Drawing for the job (mm, zero at the part's lowest x, y, z). Round coordinates to 2 decimals unless told otherwise and drop trailing zeros. Order: outer loops, then holes, each group sorted by start corner. A loop starts at its lowest first (then second) coordinate and runs counter-clockwise, first axis right, second up. Notation, with made-up numbers: (76, 6.5) -> (113, 6.5) arc R22 ccw to (113, 45.5) -> close; hole circle Ø7 at (63.5, 27.5). An arc over 180 degrees is marked (long way). Use CSV: the item, a comma, the result in double quotes.
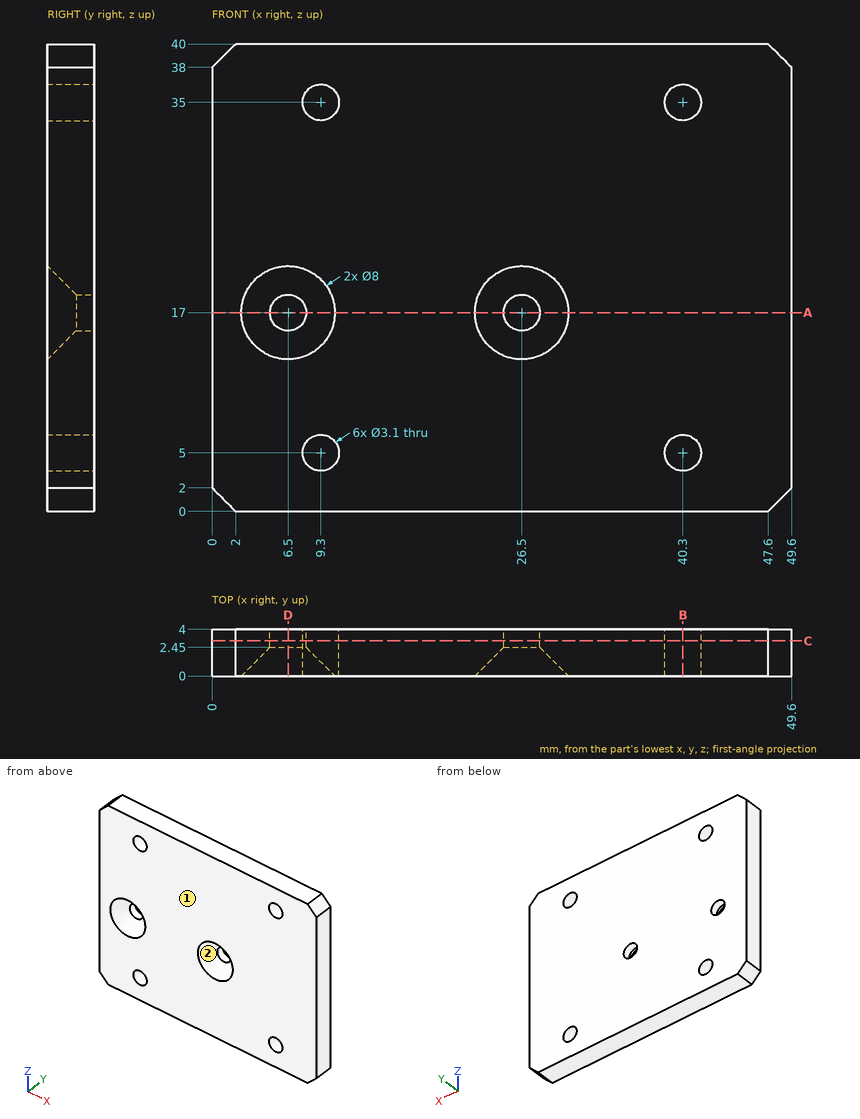
Q1. Cut at A-A (z = 17). Give the cut face in (x, y).
From the geometry:
outline,"(0, 0) -> (2.5, 0) -> (4.95, 2.45) -> (4.95, 4) -> (0, 4) -> close; (8.05, 2.45) -> (10.5, 0) -> (22.5, 0) -> (24.95, 2.45) -> (24.95, 4) -> (8.05, 4) -> close; (28.05, 2.45) -> (30.5, 0) -> (49.6, 0) -> (49.6, 4) -> (28.05, 4) -> close"
Q2. Cut at B-B (x = 40.3). Give the cut face in (y, z), plus the area to 3 significant figures.
From the geometry:
outline,"(0, 0) -> (4, 0) -> (4, 3.45) -> (0, 3.45) -> close; (0, 6.55) -> (4, 6.55) -> (4, 33.45) -> (0, 33.45) -> close; (0, 36.55) -> (4, 36.55) -> (4, 40) -> (0, 40) -> close"
area,"135 mm²"
Q3. Mould opens along Z. For the marked faces 1 and 2 say: +Z half, -Z half, draft (parallel to the pull), parting line (faces both ways), or undercut.
From the geometry:
face 1,"draft"
face 2,"undercut"
Q4. Pin check, flat tip, straight feed: pin 1 (3 mm diameter, centred on x = 26.5, z = 17, fed in from -Y). Stop position of the tip, or through.
From the geometry:
pin 1,"passes through"
Q5. Probe line 1 along Z through (x, y) = (9.3, 1.9); line 2 along X through (y, z) = (3.65, 17); line 3 along Z through (x, y) = (6.5, 3.25). List the from-to ranges inside material, lowest first.
From the geometry:
line 1,"z = 0 to 3.45, 6.55 to 33.45, 36.55 to 40"
line 2,"x = 0 to 4.95, 8.05 to 24.95, 28.05 to 49.6"
line 3,"z = 0 to 15.45, 18.55 to 40"
Q6. Cut at D-D (x = 6.5). Give the cut face in (y, z), plus the area to 3 significant figures.
From the geometry:
outline,"(0, 0) -> (4, 0) -> (4, 15.45) -> (2.45, 15.45) -> (0, 13) -> close; (0, 21) -> (2.45, 18.55) -> (4, 18.55) -> (4, 40) -> (0, 40) -> close"
area,"142 mm²"
Q7. Cut at C-C (y = 3). Give the cut face in (x, z).
From the geometry:
outline,"(0, 2) -> (2, 0) -> (47.6, 0) -> (49.6, 2) -> (49.6, 38) -> (47.6, 40) -> (2, 40) -> (0, 38) -> close; hole circle Ø3.1 at (6.5, 17); hole circle Ø3.1 at (9.3, 5); hole circle Ø3.1 at (9.3, 35); hole circle Ø3.1 at (26.5, 17); hole circle Ø3.1 at (40.3, 5); hole circle Ø3.1 at (40.3, 35)"
